Input: dimensioned drawing with shaded views. Units: mm. Origin: part minimum x, y, z. A direction names the side the tool comes from. Give positions to 0.01 mm unless a question says otherwise; leave off trailing zeros. Order: outer loops, then holes, each group sorted by start corner. A loop starts at its lowest first (then second) coordinate and runs counter-clockwise, first axis right, second up. Notation, with made-up numbers: (-31, 35.25) -> (26, 35.25) arc R33 ccw to (26, 67.25) -> close; hole circle Ø3 at (-13.75, -14). An arc over 180 degrees is marked (long way). One line per question, with ' | ' between items. Start each with the question number.
(1) Section D-D (y = 2.1). Return loops of the section in (x, z) (1 decimal), then the cut area to 3 significant figures.
(2) Set-up query: the marked faces 4 and 5. Return all of +Z, -Z, +X, -X, +Y, -Y with unobstructed straight access to the full face (end or side cutting, diameter ignored); none if empty.
(3) Section A-A (z = 10). Return loops of the section in (x, y) (1 decimal).
(4) Section B-B (x = 7). Return loops of the section in (y, z) (1 decimal).
(5) First-contact query: pin 1 Ø2.5 at (x, z) = (15.73, 22.62) entering from -Y; pin 2 Ø0.6 at (x, y) = (3, 1.5) entering from +Z. Flat tips, straight axial feed; report the tip coordinate or a pass-through.
(6) Section C-C (z = 18.5). Return loops of the section in (x, y) (1 decimal).
(7) Ray query, L1, parallel to X at y = 0.3, z = 9.5; L2, parallel to Z at x = 13, y = 2 (1 decimal); L3, parallel to Z at x = 15.5, y = 2.8 (1 decimal). Return the intervals inside material, ascending.
(8) Mould query, pull axis X, two halves, no side actions, for the marked faces 1, 2 and 3. Classes: +X half, -X half, draft (parallel to the pull), parting line (faces both ways), or undercut.
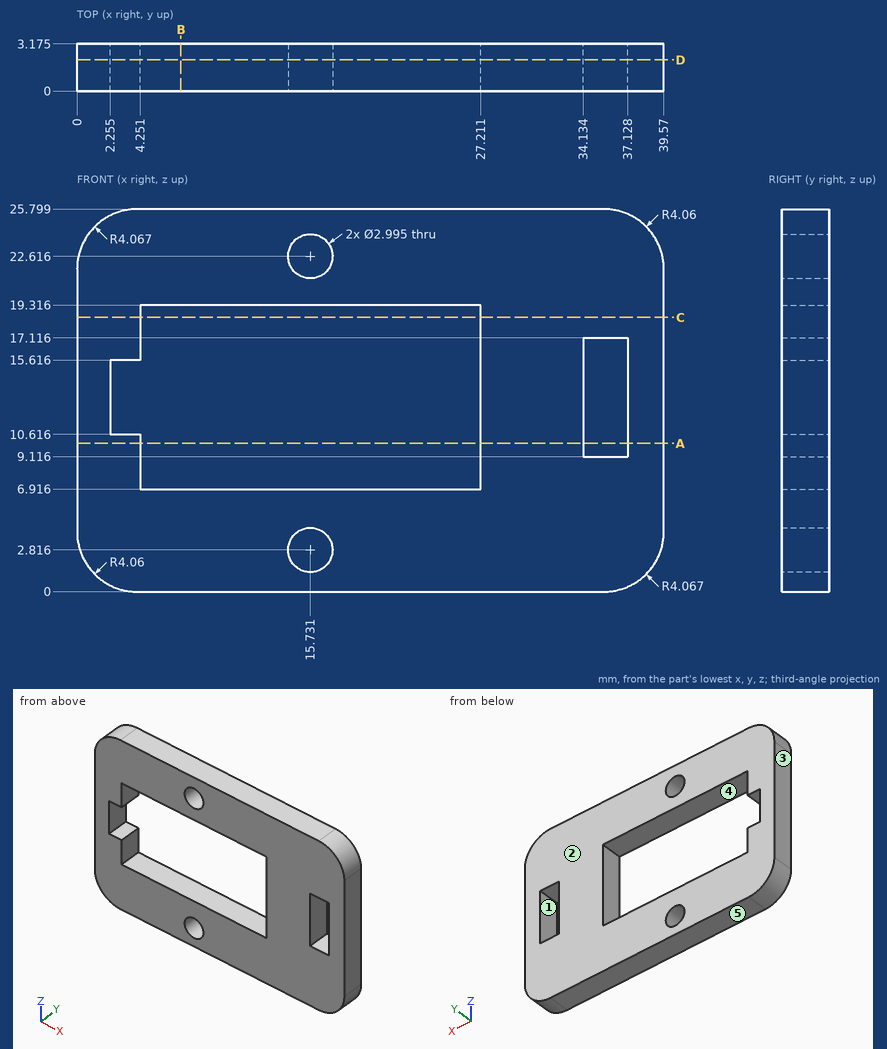
Response:
1) outline: (0, 4.1) arc R4.1 ccw to (4.1, 0) -> (35.5, 0) arc R4.1 ccw to (39.6, 4.1) -> (39.6, 21.7) arc R4.1 ccw to (35.5, 25.8) -> (4.1, 25.8) arc R4.1 ccw to (0, 21.7) -> close; hole (2.3, 10.6) -> (4.3, 10.6) -> (4.3, 6.9) -> (27.2, 6.9) -> (27.2, 19.3) -> (4.3, 19.3) -> (4.3, 15.6) -> (2.3, 15.6) -> close; hole circle Ø3 at (15.7, 2.8); hole circle Ø3 at (15.7, 22.6); hole (34.1, 9.1) -> (37.1, 9.1) -> (37.1, 17.1) -> (34.1, 17.1) -> close | area: 674 mm^2
2) face 4: +Y, -Y | face 5: -Z, +X, -X, +Y, -Y
3) outline: (0, 0) -> (4.3, 0) -> (4.3, 3.2) -> (0, 3.2) -> close; (27.2, 0) -> (34.1, 0) -> (34.1, 3.2) -> (27.2, 3.2) -> close; (37.1, 0) -> (39.6, 0) -> (39.6, 3.2) -> (37.1, 3.2) -> close
4) outline: (0, 0) -> (3.2, 0) -> (3.2, 6.9) -> (0, 6.9) -> close; (0, 19.3) -> (3.2, 19.3) -> (3.2, 25.8) -> (0, 25.8) -> close
5) pin 1: passes through | pin 2: stops at z = 25.73
6) outline: (0, 0) -> (4.3, 0) -> (4.3, 3.2) -> (0, 3.2) -> close; (27.2, 0) -> (39.6, 0) -> (39.6, 3.2) -> (27.2, 3.2) -> close
7) L1: x = 0 to 4.25, 27.21 to 34.13, 37.13 to 39.57 | L2: z = 0 to 6.9, 19.3 to 25.8 | L3: z = 0 to 1.3, 4.3 to 6.9, 19.3 to 21.1, 24.1 to 25.8
8) face 1: undercut | face 2: draft | face 3: -X half
